Design review of the part built by this model. Coordinates are the model's own, in mm. A direction names the side the tool comes from. Round coordinates to 2 decimals unless told otherwise and drop trailing zeros. Order: outer loops, then holes, each group sorted by start corner. A loop starts at its lowest first (then second) coordinate and runs counter-clockwise, first axis right, second up.
from build123d import *

# Parameters (mm, degrees)
ESQUISSE1_W        = 160
ESQUISSE1_H        = 36
ESQUISSE1_R        = 5
ESQUISSE1_W_2      = 5
ESQUISSE1_H_2      = 5
BOSS_EXTRU_1_DEPTH = 5
CONG_1_R           = 5


with BuildPart() as part:
    # Esquisse1 → Boss.-Extru.1 (new body)
    with BuildSketch(Plane.XY):
        Rectangle(ESQUISSE1_W, ESQUISSE1_H)
        Circle(ESQUISSE1_R, mode=Mode.SUBTRACT)
        with Locations((12, 0)):
            Circle(ESQUISSE1_R, mode=Mode.SUBTRACT)
        with Locations((0, 12)):
            Circle(ESQUISSE1_R, mode=Mode.SUBTRACT)
        with Locations((74.5, 7.5)):
            Rectangle(ESQUISSE1_W_2, ESQUISSE1_H_2, mode=Mode.SUBTRACT)
        with Locations((74.5, -7.5)):
            Rectangle(ESQUISSE1_W_2, ESQUISSE1_H_2, mode=Mode.SUBTRACT)
        with Locations((-74.5, 7.5)):
            Rectangle(ESQUISSE1_W_2, ESQUISSE1_H_2, mode=Mode.SUBTRACT)
        with Locations((-74.5, -7.5)):
            Rectangle(ESQUISSE1_W_2, ESQUISSE1_H_2, mode=Mode.SUBTRACT)
    extrude(amount=BOSS_EXTRU_1_DEPTH)

    # Congé1
    cong_1_edges = [part.edges().sort_by_distance(p)[0] for p in [
        (-80, 18, 2.5),
        (80, 18, 2.5),
        (80, -18, 2.5),
        (-80, -18, 2.5),
    ]]
    fillet(cong_1_edges, radius=CONG_1_R)


solid = part.part
1) Take a section at A-A on y = -3. Give the boundary of the cut face in (x, z), plus the area to 3 significant figures.
Results:
outline: (-80, 0) - (-4, 0) - (-4, 5) - (-80, 5) - close; (4, 0) - (8, 0) - (8, 5) - (4, 5) - close; (16, 0) - (80, 0) - (80, 5) - (16, 5) - close
area: 720 mm2
2) Take a section at C-C on x = 12. Give the boundary of the cut face in (y, z), plus the area to 3 significant figures.
Results:
outline: (-18, 0) - (-5, 0) - (-5, 5) - (-18, 5) - close; (5, 0) - (18, 0) - (18, 5) - (5, 5) - close
area: 130 mm2
3) For faces 1 (the face through (74, -10, 2)), 2 (the face through (-1, -8, 5)), list the 3-axis set-ups (+Z, -Z, +X, -X, +Y, -Y) from which the entire face can be reached by the end or side of a thin tool; tool diameter is ignored.
Results:
face 1: +Z, -Z
face 2: +Z, +X, -X, +Y, -Y
4) The part is to be moulded in two halves that separate along X. For faces 3 (the face through (78, 17, 3)), 4 (the face through (72, 7, 2)), 5 (the face through (-79, 16, 3)), 6 (the face through (-1, -8, 0)), say which applies: released by +X, released by -X, zero draft, split by the parting line, or undercut.
Results:
face 3: released by +X
face 4: undercut
face 5: released by -X
face 6: zero draft
5) To check wall thickness, follow line 1 along Y through (x, z) = (0, 3.4); line 2 along X through (y, z) = (9, 1.85); line 3 along X through (y, z) = (-8, 3.25). State the ranges of each line that lie inside material, in increasing order.
Results:
line 1: y = -18 to -5, 5 to 7, 17 to 18
line 2: x = -80 to -77, -72 to -4, 4 to 72, 77 to 80
line 3: x = -80 to -77, -72 to 72, 77 to 80
6) Clearance check with flat-ended pins moving along their axes: P1, Ø1.5, axis at y = -14.5, z = 4, coming from the -X side; P2, Ø4, axis at x = -4.5, y = 3, coming from the -Z side; P3, Ø6, axis at x = 0, y = 0, coming from the -Z side. State where each tip first meets the part, or that it passes through.
Results:
P1: stops at x = -79.94
P2: stops at z = 0
P3: passes through
7) Take a section at B-B on z = 2.85. Give the boundary of the cut face in (x, y), plus the area to 3 significant figures.
Results:
outline: (-80, -13) arc R5 ccw to (-75, -18) - (75, -18) arc R5 ccw to (80, -13) - (80, 13) arc R5 ccw to (75, 18) - (-75, 18) arc R5 ccw to (-80, 13) - close; hole (-77, -10) - (-72, -10) - (-72, -5) - (-77, -5) - close; hole (-77, 5) - (-72, 5) - (-72, 10) - (-77, 10) - close; hole circle Ø10 at (0, 0); hole circle Ø10 at (0, 12); hole circle Ø10 at (12, 0); hole (72, -10) - (77, -10) - (77, -5) - (72, -5) - close; hole (72, 5) - (77, 5) - (77, 10) - (72, 10) - close
area: 5,400 mm2
